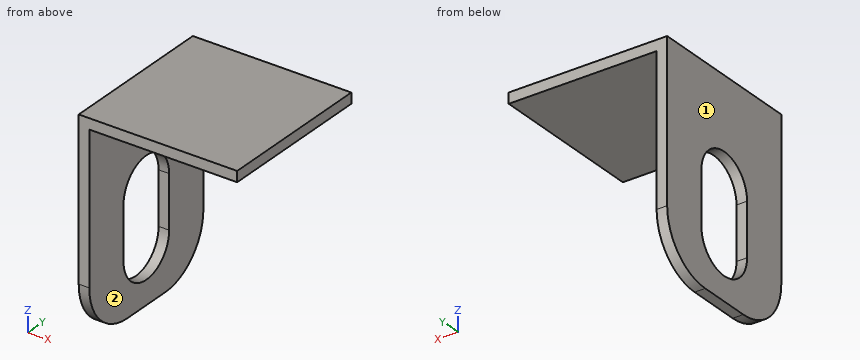
```python
from build123d import *

# Parameters (mm, degrees)
SKETCH_1_W               = 2
SKETCH_1_H               = 40
SKETCH_1_W_2             = 28
SKETCH_1_H_2             = 2
EXTRUDE_1_DEPTH          = 15
FILLET_1_R               = 10
CUT_EXTRUDE_1_DEPTH      = 38.536648758
CUT_EXTRUDE_1_DEPTH_BACK = 38.536648758


with BuildPart() as part:
    # 草图1 → 凸台-拉伸1 (new, symmetric)
    with BuildSketch(Plane(origin=(0, 0, 0), x_dir=(1, 0, 0), z_dir=(0, 1, 0))):
        Rectangle(SKETCH_1_W, SKETCH_1_H)
        with Locations((15, -19)):
            Rectangle(SKETCH_1_W_2, SKETCH_1_H_2)
    extrude(amount=EXTRUDE_1_DEPTH, both=True)

    # 圆角1
    fillet_1_edges = [part.edges().sort_by_distance(p)[0] for p in [
        (0, 15, -20),
        (0, -15, -20),
    ]]
    fillet(fillet_1_edges, radius=FILLET_1_R)

    # 草图2 → 切除-拉伸1 (cut, two sides: drawn at the far end of the back side and taken through both)
    with BuildSketch(Plane(origin=(1, 0, 0), x_dir=(0, 0, -1), z_dir=(1, 0, 0)).offset(-CUT_EXTRUDE_1_DEPTH_BACK)):
        with BuildLine():
            Line((-0.5, 6), (9.5, 6))
            ThreePointArc((9.5, 6), (15.5, 0), (9.5, -6))
            Line((9.5, -6), (-0.5, -6))
            ThreePointArc((-0.5, -6), (-6.5, 0), (-0.5, 6))
        make_face()
    extrude(amount=CUT_EXTRUDE_1_DEPTH + CUT_EXTRUDE_1_DEPTH_BACK, mode=Mode.SUBTRACT)


solid = part.part
```
The listing builds one solid part. Answer for the finished solid, in the listing's coordinates (mm). Face numbers are marked on the shaded views. A direction names the side the tool comes from. Give positions to 0.01 mm unless a question says otherwise; leave off trailing zeros. Write each loop counter-clockwise with the first axis right and the second up, starting at its lowest first coordinate (ties: lowest second). Pieces come first, ordered by that corner, then holes. Notation, with made-up numbers: (-18, 47.25) -> (41, 47.25) arc R17 ccw to (41, 56.25) -> close; hole circle Ø7 at (78.25, 50). An arc over 180 degrees is marked (long way). Write item = value, one per line. Start each with the question number.
1) The part is cut by section A-A, the plane y = 0. Determine the outline of the cut face in (x, z), and give its area (3 significant figures).
2) Which of the six approach directions +Z, -Z, +X, -X, +Y, -Y give full straight-line access (tool end or side, diameter ignored) to the marked faces 1 and 2?
3) The part is cut by section C-C, the plane z = -14. Determine the outline of the cut face in (x, y).
4) Each of these flat-tipped pins is pushed along its axis until it touches: pin 1 (14 mm diameter, centred on x = 9.5, y = -4.5, fed in from -Z); pin 2 (10 mm diameter, centred on y = -6.5, z = -12, fed in from +X). Where does it stop, or does it pass through?
5) The part is cut by section B-B, the plane z = -0.5. Determine the outline of the cut face in (x, y).
6) Straight lines are drawn through the part: line 1 along X through (y, z) = (13, 3); line 2 along Z through (x, y) = (10.5, 1.5). For each, find the intervals that lie inside material, in ascending order.
7) The part is cut by section D-D, the plane x = 26.5. Determine the outline of the cut face in (y, z).
Solutions:
q1.outline = (-1, -20) -> (1, -20) -> (1, -15.5) -> (-1, -15.5) -> close; (-1, 6.5) -> (1, 6.5) -> (1, 18) -> (29, 18) -> (29, 20) -> (-1, 20) -> close
q1.area = 92.0 mm²
q2.face_1 = +Z, -Z, -X, +Y, -Y
q2.face_2 = -Z, +X, +Y, -Y
q3.outline = (-1, -14.17) -> (1, -14.17) -> (1, -3.97) -> (-1, -3.97) -> close; (-1, 3.97) -> (1, 3.97) -> (1, 14.17) -> (-1, 14.17) -> close
q4.pin_1 = 18
q4.pin_2 = 1
q5.outline = (-1, -15) -> (1, -15) -> (1, -6) -> (-1, -6) -> close; (-1, 6) -> (1, 6) -> (1, 15) -> (-1, 15) -> close
q6.line_1 = -1 to 1
q6.line_2 = 18 to 20
q7.outline = (-15, 18) -> (15, 18) -> (15, 20) -> (-15, 20) -> close
